from build123d import *

# Parameters (mm, degrees)
BOSS_EXTRUDE1_DEPTH = 56
FILLET1_R           = 10
SKETCH15_R          = 16
CUT_EXTRUDE1_DEPTH  = 73.567889266


with BuildPart() as part:
    # Sketch1 → Boss-Extrude1 (new body)
    with BuildSketch(Plane(origin=(0, 0, 0), x_dir=(0, 0, -1), z_dir=(1, 0, 0))):
        Polygon((44.245922439, 12.13), (34.245922439, 12.13), (34.245922439, 8.8), (44.245922439, 8.8), (44.245922439, 6.8), (30.245922439, 6.8), (25.379144578, 1), (17.228544282, 1), (28.245922439, 14.13), (44.245922439, 14.13), align=None)
    extrude(amount=BOSS_EXTRUDE1_DEPTH)

    # Fillet1
    fillet1_edges = [part.edges().sort_by_distance(p)[0] for p in [
        (28, 6.8, -30.245922439),
    ]]
    fillet(fillet1_edges, radius=FILLET1_R)

    # Sketch15 → Cut-Extrude1 (cut, through all)
    with BuildSketch(Plane(origin=(0, 14.13, 0), x_dir=(1, 0, 0), z_dir=(0, 1, 0))):
        with Locations((28, 44.245922439)):
            Circle(SKETCH15_R)
    extrude(amount=-CUT_EXTRUDE1_DEPTH, mode=Mode.SUBTRACT)


solid = part.part
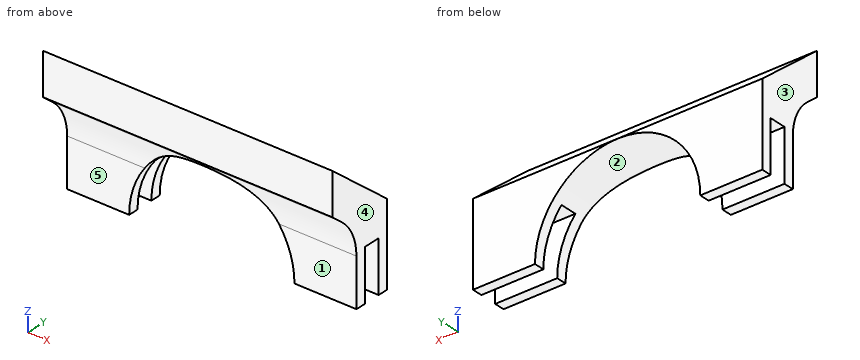
Geometry check sheet. Reference: the model listing, model coordinates, mm. Face numbers are marked on the shaded views. A direction names the side the tool comes from. Coordinates: 2 decimals unless noted, no trailing zeros. Order: outer loops, then holes, each group sorted by start corner. A loop starts at its lowest first (then second) coordinate and runs counter-clockwise, first axis right, second up. Notation, with made-up numbers: (11, 42.25) - (59, 42.25) arc R33 ccw to (59, 77.25) - close; hole circle Ø2 at (79, -23). An arc over 180 degrees is marked (long way). Answer in a Markdown table with one row per item. Add a question column.
1) Cross-section at C-C, the plane z = -33.5. Record the cut outline in (x, y).
2) Gauge pin test, flat ends, axial feed: P1, Ø1.7, axis at x = 48.5, y = 11, coming from the -Z side; P2, Ø1.5, axis at x = 39, y = 10, coming from the -Z side; P3, Ø7.5, axis at x = 10, z = -37.5, coming from the -Y side; P4, Ø3.5, axis at x = 6, y = 10, coming from the -Z side. Record the tip position at first contact, or that the pin passes through.
3) Cross-section at A-A, the plane x = 11. Record the cut outline in (y, z).
4) Cross-section at D-D, the plane y = 10. Record the cut outline in (x, z).
5) Cross-section at B-B, the plane z = -41. Record the cut outline in (x, y), then the cut area to 3 significant figures.
6) Release check for a two-part mould opening along X. For the marked faces 1, 2 and 3 record: +X half, -X half, draft (parallel to the pull), parting line (faces both ways), or undercut.
7) Set-up check for the marked faces 4 and 5: record each of +Z, -Z, +X, -X, +Y, -Y from which the full face is reachable in a straight line by a thin tool's end or side.
8) Material ranges on line 1 along Y through (x, z) = (53.5, -41.5); line 2 along Y through (x, z) = (33, -28.25); line 3 along X through (y, z) = (12.25, -31.25), recorded low to high. Write a range as [from, to].
Check result:
| question | item | result |
|---|---|---|
| 1 | outline | (0, 6.7) - (16.15, 6.7) - (16.15, 14.13) - (0, 14.13) - close; (39.85, 6.7) - (56, 6.7) - (56, 14.13) - (39.85, 14.13) - close |
| 2 | P1 | stops at z = -34.25 |
| 2 | P2 | stops at z = -33.39 |
| 2 | P3 | stops at y = 6.73 |
| 2 | P4 | stops at z = -44.25 |
| 3 | outline | (1, -25.38) - (3.23, -27.25) arc R10 cw to (6.8, -34.91) - (6.8, -44.25) - (8.8, -44.25) - (8.8, -34.25) - (12.13, -34.25) - (12.13, -44.25) - (14.13, -44.25) - (14.13, -28.25) - (1, -17.23) - close |
| 4 | outline | (0, -34.25) - (15.51, -34.25) arc R16 cw to (40.49, -34.25) - (56, -34.25) - (56, -24.78) - (0, -24.78) - close |
| 5 | outline | (0, 6.8) - (12.33, 6.8) - (12.33, 8.8) - (0, 8.8) - close; (0, 12.13) - (12.33, 12.13) - (12.33, 14.13) - (0, 14.13) - close; (43.67, 6.8) - (56, 6.8) - (56, 8.8) - (43.67, 8.8) - close; (43.67, 12.13) - (56, 12.13) - (56, 14.13) - (43.67, 14.13) - close |
| 5 | area | 98.7 mm² |
| 6 | face 1 | draft |
| 6 | face 2 | undercut |
| 6 | face 3 | -X half |
| 7 | face 4 | +Z, -Z, +X, +Y, -Y |
| 7 | face 5 | -Z, +X, -X, -Y |
| 8 | line 1 | y = [6.8, 8.8], [12.13, 14.13] |
| 8 | line 2 | y = [4.26, 14.13] |
| 8 | line 3 | x = [0, 18.67], [37.33, 56] |
